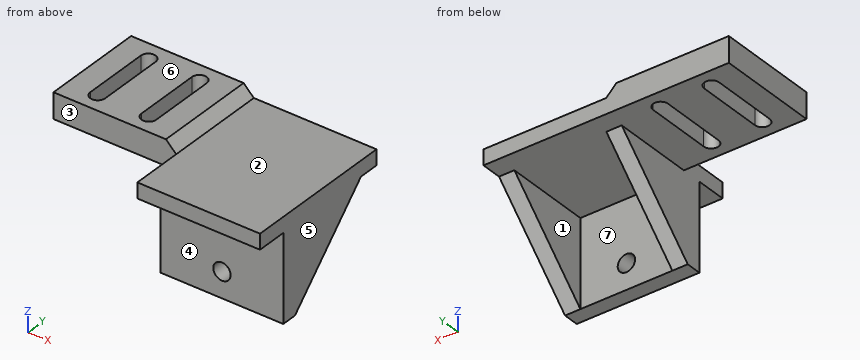
from build123d import *

# Parameters (mm, degrees)
F1_DEPTH  = 48
F2_DEPTH  = 3
F3_W      = 24
F3_H      = 10
F4_DEPTH  = 25
F6_DEPTH  = 3
F7_R      = 1.7
F8_DEPTH  = 9.001
F10_DEPTH = 20
F12_DEPTH = 22.001


with BuildPart() as f1:
    # F0 (on Right) → F1 (new body)
    with BuildSketch(Plane.YZ):
        Polygon((24, 20), (-6, 20), (-6, 17), (0, 17), (0, 0), (3, 0), (3, 17), (20, 17), (24, 17), align=None)
    extrude(amount=-F1_DEPTH)

    # F0 (on Right) → F2 (join)
    with BuildSketch(Plane.YZ):
        Polygon((3, 0), (20, 17), (3, 17), align=None)
    extrude(amount=-F2_DEPTH)

    # F3 (on face) → F4 (cut)
    with BuildSketch(Plane.XY.offset(20)):
        with Locations((-36, -1)):
            Rectangle(F3_W, F3_H)
    extrude(amount=-F4_DEPTH, mode=Mode.SUBTRACT)

    # F5 (on face) → F6 (join)
    with BuildSketch(Plane(origin=(-24, 0, 0), x_dir=(0, -1, 0), z_dir=(-1, 0, 0))):
        Polygon((-3, 0), (-3, 17), (-20, 17), align=None)
    extrude(amount=-F6_DEPTH)

    # F7 (on face) → F8 (cut, through all)
    with BuildSketch(Plane(origin=(0, 3, 0), x_dir=(-1, 0, 0), z_dir=(0, 1, 0))):
        with Locations((12, 5)):
            Circle(F7_R)
    extrude(amount=-F8_DEPTH, mode=Mode.SUBTRACT)

    # F9 (on face) → F10 (join)
    with BuildSketch(Plane.XZ.offset(-4)):
        Polygon((-48, 20), (-24, 20), (-26, 22), (-48, 22), align=None)
    extrude(amount=-F10_DEPTH)

    # F11 (on face) → F12 (cut, through all)
    with BuildSketch(Plane.XY.offset(22)):
        with BuildLine():
            Line((-40.55, 7.5), (-40.55, 20.5))
            ThreePointArc((-40.55, 20.5), (-42, 21.95), (-43.45, 20.5))
            Line((-43.45, 20.5), (-43.45, 7.5))
            ThreePointArc((-43.45, 7.5), (-42, 6.05), (-40.55, 7.5))
        make_face()
        with BuildLine():
            Line((-30.55, 7.5), (-30.55, 20.5))
            ThreePointArc((-30.55, 20.5), (-32, 21.95), (-33.45, 20.5))
            Line((-33.45, 20.5), (-33.45, 7.5))
            ThreePointArc((-33.45, 7.5), (-32, 6.05), (-30.55, 7.5))
        make_face()
    extrude(amount=-F12_DEPTH, mode=Mode.SUBTRACT)


solid = f1.part
Can you work these out from the model? Positions are in its coordinate system, mm. Face numbers are marked on the shaded views. A direction names the side the tool comes from. Round coordinates to 2 decimals unless told otherwise and drop trailing zeros. Write each loop counter-clockwise with the first axis right and the second up, starting at its lowest first coordinate (ties: lowest second). Pieces come first, ordered by that corner, then holes. Notation, with made-up numbers: (80, 19) -> (134, 19) arc R18 cw to (134, 25) -> close; hole circle Ø2 at (-30.75, 45.5). An arc over 180 degrees is marked (long way). One line per question, with ' | ' between items. Start each with the question number.
1) Suppose I cut it at A-A on y = 9. Write out the boundary of the cut face in (x, z), then the cut area to 3 significant figures.
2) I'm going to push flat-ended pins straight in: P1, Ø3, axis at y = 0.5, z = 14, coming from the -X side; P2, Ø4, axis at x = -12, z = 5, coming from the +Y side; P3, Ø1.8, axis at x = -17.5, y = -3, coming from the -Z side; P4, Ø10, axis at x = -34, z = 7.5, coming from the -Y side. Where does each tip first touch, or does it pass through?
3) Suppose I cut it at D-D on x = -6. Write out the boundary of the cut face in (y, z), then the cut area to 3 significant figures.
4) Suppose I cut it at B-B on x = -12. Write out the boundary of the cut face in (y, z), then the cut area to 3 significant figures.
5) On a 3-axis mill with a long thin cutter (end or side, diameter ignored), from which of +Z, -Z, +X, -X, +Y, -Y can I reach the whole of each face in a straight line? I mean the marked faces 1, 2, 3 and 4. Say none if no direction works.
6) Suppose I cut it at C-C on z = 5. Write out the boundary of the cut face in (x, y), then the cut area to 3 significant figures.
7) I need wall thicknesses on line 1 (Z direction, x = -12, y = 2); line 2 (Y direction, x = -16, z = 1.5); line 3 (X direction, y = 9.5, z = 11.75). Which ranges of each line are inside material? Lowest first, please. Write a range as [from, to].
8) If we mould it in two halves opening along X, with no side actions, what happens to the marked faces 5, 6 and 7? For each: released by +X, released by -X, zero draft, split by the parting line, or undercut.
Return value:
1) outline: (-48, 17) -> (-43.45, 17) -> (-43.45, 22) -> (-48, 22) -> close; (-40.55, 17) -> (-33.45, 17) -> (-33.45, 22) -> (-40.55, 22) -> close; (-30.55, 17) -> (-24, 17) -> (-24, 6) -> (-21, 6) -> (-21, 17) -> (-3, 17) -> (-3, 6) -> (0, 6) -> (0, 20) -> (-24, 20) -> (-26, 22) -> (-30.55, 22) -> close | area: 227 mm2
2) P1: stops at x = -24 | P2: stops at y = 3 | P3: stops at z = 17 | P4: passes through
3) outline: (-6, 17) -> (0, 17) -> (0, 0) -> (3, 0) -> (3, 17) -> (24, 17) -> (24, 20) -> (-6, 20) -> close | area: 141 mm2
4) outline: (-6, 17) -> (0, 17) -> (0, 6.7) -> (3, 6.7) -> (3, 17) -> (24, 17) -> (24, 20) -> (-6, 20) -> close; (0, 0) -> (3, 0) -> (3, 3.3) -> (0, 3.3) -> close | area: 131 mm2
5) face 1: -Z, +Y | face 2: +Z, +X, +Y, -Y | face 3: +Z, -Z, -X, -Y | face 4: -Z, +X, -X, -Y
6) outline: (-24, 0) -> (-13.7, 0) -> (-13.7, 3) -> (-21, 3) -> (-21, 8) -> (-24, 8) -> close; (-10.3, 0) -> (0, 0) -> (0, 8) -> (-3, 8) -> (-3, 3) -> (-10.3, 3) -> close | area: 91.8 mm2
7) line 1: z = [0, 3.3], [6.7, 20] | line 2: y = [0, 3] | line 3: x = [-24, -21], [-3, 0]
8) face 5: released by +X | face 6: zero draft | face 7: undercut
